The listing builds one solid part. Answer for the finished solid, in the listing's coordinates (mm). Coordinates: 2 decimals unless noted, no trailing zeros. Write each loop counter-clockwise with the first axis right and the second up, starting at its lowest first coordinate (ties: lowest second). Pieces come first, ordered by that corner, then holes.
from build123d import *

# Parameters (mm, degrees)
SKETCH1_W           = 10
SKETCH1_H           = 70
BOSS_EXTRUDE1_DEPTH = 1.5
SKETCH3_W           = 0.2
SKETCH3_H           = 60
CUT_EXTRUDE2_DEPTH  = 10
SKETCH4_W           = 6
SKETCH4_H           = 1.5
CUT_EXTRUDE3_DEPTH  = 10


with BuildPart() as part:
    # Sketch1 → Boss-Extrude1 (new body)
    with BuildSketch(Plane(origin=(0, 0, 0), x_dir=(0, 0, -1), z_dir=(1, 0, 0))):
        with Locations((-5, 4.155844156)):
            Rectangle(SKETCH1_W, SKETCH1_H)
    extrude(amount=BOSS_EXTRUDE1_DEPTH)

    # Sketch3 → Cut-Extrude2 (cut)
    with BuildSketch(Plane(origin=(1.5, 0, 0), x_dir=(0, 0, -1), z_dir=(1, 0, 0))):
        with Locations((-5, 4.155844156)):
            Rectangle(SKETCH3_W, SKETCH3_H)
    extrude(amount=-CUT_EXTRUDE2_DEPTH, mode=Mode.SUBTRACT)

    # Sketch4 → Cut-Extrude3 (cut)
    with BuildSketch(Plane(origin=(1.5, 0, 0), x_dir=(0, 0, -1), z_dir=(1, 0, 0))):
        with Locations((-5, 38.405844156)):
            Rectangle(SKETCH4_W, SKETCH4_H)
        with Locations((-5, -30.094155844)):
            Rectangle(SKETCH4_W, SKETCH4_H)
    extrude(amount=-CUT_EXTRUDE3_DEPTH, mode=Mode.SUBTRACT)


solid = part.part
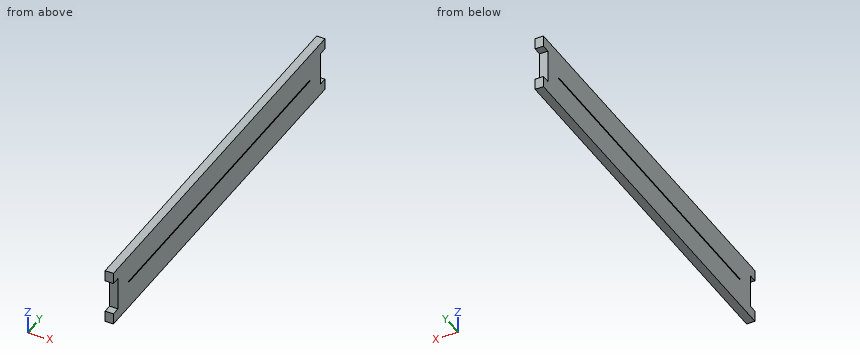
Q1. Given pin 1 (0.8 mm diameter, centred on x = 1, z = 4, fed in from -Y), flat-ended and moving along its own axis, determine where the tip first touches the part or whether it passes through.
Answers below:
pin 1: stops at y = -29.34
Q2. The part is cut by section A-A, the plane y = -8.5. Write down the section's boundary in (x, z), then the cut area to 3 significant figures.
Answers below:
outline: (0, 0) - (1.5, 0) - (1.5, 4.9) - (0, 4.9) - close; (0, 5.1) - (1.5, 5.1) - (1.5, 10) - (0, 10) - close
area: 14.7 mm2
Q3. The part is cut by section C-C, the plane z = 4.25. Write down the section's boundary in (x, y).
Answers below:
outline: (0, -29.34) - (1.5, -29.34) - (1.5, 37.66) - (0, 37.66) - close
Q4. The part is cut by section B-B, the plane x = 0.85. Write down the section's boundary in (y, z), then the cut area to 3 significant figures.
Answers below:
outline: (-30.84, 0) - (39.16, 0) - (39.16, 2) - (37.66, 2) - (37.66, 8) - (39.16, 8) - (39.16, 10) - (-30.84, 10) - (-30.84, 8) - (-29.34, 8) - (-29.34, 2) - (-30.84, 2) - close; hole (-25.84, 4.9) - (34.16, 4.9) - (34.16, 5.1) - (-25.84, 5.1) - close
area: 670 mm2
Q5. Find the intervals of material crossed by probe 1 along Z at (x, y) = (0.2, -3); probe 2 along Y at (x, z) = (1.2, 2.75), in increasing order.
Answers below:
probe 1: z = 0 to 4.9, 5.1 to 10
probe 2: y = -29.34 to 37.66
